The listing builds one solid part. Answer for the finished solid, in the listing's coordinates (mm). A direction names the side the tool comes from. Round coordinates to 2 decimals unless told otherwise and drop trailing zeros. Write each loop counter-clockwise with the first axis right and the second up, starting at its lowest first coordinate (ties: lowest second). Pieces come first, ordered by that corner, then holes. Notation, with made-up numbers: (46.25, 67.5) - (75.25, 67.5) arc R22 cw to (75.25, 81.5) - close; hole circle Ø9 at (-21.75, -10.75). An arc over 180 degrees is marked (long way). Answer in a Markdown table with one row per item.
from build123d import *

# Parameters (mm, degrees)
BASE_FLANGE2_DEPTH           = 5
EDGE_FLANGE3_STRIP_W         = 26
EDGE_FLANGE3_STRIP_H         = 5
EDGE_FLANGE3_STRIP_CUT_DEPTH = 120
EDGE_FLANGE3_DEPTH           = 120
SKETCH18_R                   = 4
CUT_EXTRUDE1_DEPTH           = 10


# Sheet-metal steps are written as plain solids
with BuildPart() as part:
    # Sketch1 → Base-Flange2 (new body)
    with BuildSketch(Plane.XY):
        with BuildLine():
            Line((60, 66.5), (60, 100.5))
            ThreePointArc((60, 100.5), (58.242640687, 104.742640687), (54, 106.5))
            Line((54, 106.5), (-54, 106.5))
            ThreePointArc((-54, 106.5), (-58.242640687, 104.742640687), (-60, 100.5))
            Line((-60, 100.5), (-60, 66.5))
            Line((-60, 66.5), (60, 66.5))
        make_face()
    extrude(amount=BASE_FLANGE2_DEPTH)

    # Edge-Flange3 strip (across the edge) → Edge-Flange3 strip cut (cut)
    with BuildSketch(Plane(origin=(-60, 66.5, 5), x_dir=(0, 1, 0), z_dir=(1, 0, 0))):
        with Locations((-10, -2.5)):
            Rectangle(EDGE_FLANGE3_STRIP_W, EDGE_FLANGE3_STRIP_H)
    extrude(amount=EDGE_FLANGE3_STRIP_CUT_DEPTH, mode=Mode.SUBTRACT)

    # Edge-Flange3 section (across the edge) → Edge-Flange3 (add)
    with BuildSketch(Plane(origin=(-60, 66.5, 5), x_dir=(0, 1, 0), z_dir=(1, 0, 0))):
        with BuildLine():
            Line((-5, 3), (-5, 205))
            Line((-5, 205), (0, 205))
            Line((0, 205), (0, 3))
            ThreePointArc((0, 3), (0.878679656, 0.878679656), (3, 0))
            Line((3, 0), (3, -5))
            ThreePointArc((3, -5), (-2.656854249, -2.656854249), (-5, 3))
        make_face()
    extrude(amount=EDGE_FLANGE3_DEPTH)

    # Sketch18 → Cut-Extrude1 (cut)
    with BuildSketch(Plane(origin=(0, 66.5, 0), x_dir=(1, 0, 0), z_dir=(0, 1, 0))):
        with Locations(Location((36.205, -197, 0), (0, 0, 270))):
            Circle(SKETCH18_R)
        with Locations(Location((-36.205, -197, 0), (0, 0, 270))):
            Circle(SKETCH18_R)
        with Locations(Location((-36.205, -127, 0), (0, 0, 270))):
            Circle(SKETCH18_R)
        with Locations(Location((36.205, -127, 0), (0, 0, 270))):
            Circle(SKETCH18_R)
        with Locations(Location((36.205, -57, 0), (0, 0, 270))):
            Circle(SKETCH18_R)
        with Locations(Location((-36.205, -57, 0), (0, 0, 270))):
            Circle(SKETCH18_R)
        with Locations((-60, -197)):
            Circle(SKETCH18_R)
        with Locations((-60, -127)):
            Circle(SKETCH18_R)
        with Locations((-60, -57)):
            Circle(SKETCH18_R)
        with Locations((60, -197)):
            Circle(SKETCH18_R)
        with Locations((60, -127)):
            Circle(SKETCH18_R)
        with Locations((60, -57)):
            Circle(SKETCH18_R)
    extrude(amount=-CUT_EXTRUDE1_DEPTH, mode=Mode.SUBTRACT)


solid = part.part
(1) Flat-ended cylindrical pins translate along their axes: pin 1 (9 mm diameter, centred on x = 36.205, z = 197, fed in from +Y); pin 2 (5 mm diameter, centred on x = -36.205, z = 57, fed in from +Y); pin 3 (9 mm diameter, centred on x = -36.205, z = 127, fed in from -Y). Find the tip coordinate at first contact, or state that the pin passes through.
Checked values:
| item | result |
|---|---|
| pin 1 | stops at y = 66.5 |
| pin 2 | passes through |
| pin 3 | stops at y = 61.5 |
(2) For a pull along X with two mould halves and no side action, classify faces 1 (the flat face through (-1, 64, 210)), 2 (the flat face through (60, 64, 162)), 3 (the flat face through (-60, 65, 17)), 4 (the cylindrical face through (40.17, 64.04, 126.48)) as pulls with the +X half, pulls with the -X half, needs draft (parallel to the pull), parting line crosses it, or undercut.
Checked values:
| item | result |
|---|---|
| face 1 | needs draft |
| face 2 | pulls with the +X half |
| face 3 | pulls with the -X half |
| face 4 | undercut |
(3) Section C-C (y = 91.5) is taken. Give the vertices of the cut face in (x, z).
Checked values:
| item | result |
|---|---|
| outline | (-60, 0) - (60, 0) - (60, 5) - (-60, 5) - close |
(4) Section A-A (z = 127) is taken. Give the vertices of the cut face in (x, y) (3 decimals), and give its area (3 significant figures).
Checked values:
| item | result |
|---|---|
| outline | (-56, 61.5) - (-40.205, 61.5) - (-40.205, 66.5) - (-56, 66.5) - close; (-32.205, 61.5) - (32.205, 61.5) - (32.205, 66.5) - (-32.205, 66.5) - close; (40.205, 61.5) - (56, 61.5) - (56, 66.5) - (40.205, 66.5) - close |
| area | 480 mm2 |
(5) Find the intervals of material crossed by line 1 (X direction, y = 62, z = 197) (3 decimals); line 2 (Y direction, x = 26.5, z = 164.5); line 3 (Z direction, x = 18, y = 79), in increasing order.
Checked values:
| item | result |
|---|---|
| line 1 | x = -56 to -40.205, -32.205 to 32.205, 40.205 to 56 |
| line 2 | y = 61.5 to 66.5 |
| line 3 | z = 0 to 5 |
(6) For faces 5 (the flat face through (-1, 88, 5)), 6 (the cylindrical face through (37.406, 64.035, 200.815)), determine the directions among +Z, -Z, +X, -X, +Y, -Y from which every point of the face is accessible in a straight line to the end or side of a thin tool.
Checked values:
| item | result |
|---|---|
| face 5 | +Z, +X, -X, +Y |
| face 6 | +Y, -Y |
(7) Section B-B (x = -18) is taken. Give the vertices of the cut face in (y, z), and give its area (3 significant figures).
Checked values:
| item | result |
|---|---|
| outline | (61.5, 8) arc R8 ccw to (69.5, 0) - (106.5, 0) - (106.5, 5) - (69.5, 5) arc R3 cw to (66.5, 8) - (66.5, 210) - (61.5, 210) - close |
| area | 1,240 mm2 |
(8) Section D-D (z = 44.5) is taken. Give the vertices of the cut face in (x, y).
Checked values:
| item | result |
|---|---|
| outline | (-60, 61.5) - (60, 61.5) - (60, 66.5) - (-60, 66.5) - close |
